Input: part model. Units: mm. Frame: model coordinates. A direction names the side the tool comes from. Coordinates: 2 decimals unless noted, no trailing zeros. Loops run counter-clockwise (first coordinate to the right, second up) from the corner with the lowest first, then second, coordinate; pieces in that order, holes last.
(1) Section C-C, the plane y = 16. Return loops of the section in (x, z), then the cut area to 3 significant figures.
(2) Section D-D, the plane x = 21.5. Return loops of the section in (y, z).
(3) Section B-B, the plane x = 4. Return loops of the section in (y, z).
(4) Line query: L1, parallel to X at y = 6, z = 1.45; L2, parallel to X at y = 10, z = 1.9; L3, parallel to X at y = 73.5, z = 1.55. Output: solid intervals per line, ascending.
(5) Set-up query: faces 4 (the face through (31, 13.53, 1)), 5 (the face through (25, 3.13, 1)), 6 (the face through (21, 37.18, 1)), 7 (the face through (-24, 3.13, 1)), 8 (the face through (38.259, 12, 1)). Return all of +Z, -Z, +X, -X, +Y, -Y with unobstructed straight access to the full face (end or side cutting, diameter ignored); none if empty.
(6) Mould query, pull axis Y, two halves, no side actions, for faces 1 (the face through (-17.563, 34, 1)), 2 (the face through (20.209, 0, 1)), 3 (the face through (-0.165, 90.126, 0.986)). Classes: released by +Y, released by -Y, zero draft, split by the parting line, or undercut.
(7) Contact query for flat-ended pins moving along their axis: P1, Ø0.6, axis at x = -20.5, z = 1, coming from the -Y side; P2, Ø0.6, axis at y = 34.5, z = 1.5, coming from the -X side; P3, Ø1, axis at y = 0.5, z = 1, coming from the +X side. Output: stop coordinate, or through.
(8) Section A-A, the plane y = 5.5. Return loops of the section in (x, z), then the cut area to 3 significant figures.
```python
from build123d import *

# Parameters (mm, degrees)
SKETCH_1_R      = 9.55
SKETCH_1_R_2    = 2.55
SKETCH_1_W      = 6.1
SKETCH_1_H      = 6.1
EXTRUDE_1_DEPTH = 2
FILLET_3_R      = 1.5


with BuildPart() as part:
    # 草图1 → 凸台-拉伸1 (new body)
    with BuildSketch(Plane.XY):
        with BuildLine():
            Line((-28.741188564, 3.13029316), (-28.741188564, 7.13029316))
            Line((-28.741188564, 7.13029316), (-27.291188564, 7.13029316))
            Line((-27.291188564, 7.13029316), (-27.291188564, 10.33029316))
            Line((-27.291188564, 10.33029316), (-28.741188564, 10.33029316))
            Line((-28.741188564, 10.33029316), (-28.741188564, 13.53029316))
            Line((-28.741188564, 13.53029316), (-32.841188564, 13.53029316))
            Line((-32.841188564, 13.53029316), (-32.841188564, 10.33029316))
            Line((-32.841188564, 10.33029316), (-34.291188564, 10.33029316))
            Line((-34.291188564, 10.33029316), (-34.291188564, 7.13029316))
            Line((-34.291188564, 7.13029316), (-32.841188564, 7.13029316))
            Line((-32.841188564, 7.13029316), (-32.841188564, 3.13029316))
            Line((-32.841188564, 3.13029316), (-37.841188564, 3.13029316))
            Line((-37.841188564, 3.13029316), (-37.841188564, 20.08029316))
            Line((-37.841188564, 20.08029316), (-16.791188564, 73.13029316))
            ThreePointArc((-16.791188564, 73.13029316), (0.208811436, 90.13029316), (17.208811436, 73.13029316))
            Line((17.208811436, 73.13029316), (38.258811436, 20.08029316))
            Line((38.258811436, 20.08029316), (38.258811436, 3.13029316))
            Line((38.258811436, 3.13029316), (33.258811436, 3.13029316))
            Line((33.258811436, 3.13029316), (33.258811436, 7.13029316))
            Line((33.258811436, 7.13029316), (34.708811436, 7.13029316))
            Line((34.708811436, 7.13029316), (34.708811436, 10.33029316))
            Line((34.708811436, 10.33029316), (33.258811436, 10.33029316))
            Line((33.258811436, 10.33029316), (33.258811436, 13.53029316))
            Line((33.258811436, 13.53029316), (29.158811436, 13.53029316))
            Line((29.158811436, 13.53029316), (29.158811436, 10.33029316))
            Line((29.158811436, 10.33029316), (27.708811436, 10.33029316))
            Line((27.708811436, 10.33029316), (27.708811436, 7.13029316))
            Line((27.708811436, 7.13029316), (29.158811436, 7.13029316))
            Line((29.158811436, 7.13029316), (29.158811436, 3.13029316))
            Line((29.158811436, 3.13029316), (20.208811436, 3.13029316))
            Line((20.208811436, 3.13029316), (20.208811436, -2.86970684))
            Line((20.208811436, -2.86970684), (12.208811436, -2.86970684))
            Line((12.208811436, -2.86970684), (12.208811436, 3.13029316))
            Line((12.208811436, 3.13029316), (-11.791188564, 3.13029316))
            Line((-11.791188564, 3.13029316), (-11.791188564, -2.86970684))
            Line((-11.791188564, -2.86970684), (-19.791188564, -2.86970684))
            Line((-19.791188564, -2.86970684), (-19.791188564, 3.13029316))
            Line((-19.791188564, 3.13029316), (-28.741188564, 3.13029316))
        make_face()
        with Locations((0.208811436, 73.13029316)):
            Circle(SKETCH_1_R, mode=Mode.SUBTRACT)
        with Locations((-4.791188564, 28.13029316)):
            Circle(SKETCH_1_R_2, mode=Mode.SUBTRACT)
        with Locations(Location((5.208811436, 28.13029316, 0), (0, 0, 180))):
            Circle(SKETCH_1_R_2, mode=Mode.SUBTRACT)
        with Locations((-20.612527992, 34.13029316)):
            Rectangle(SKETCH_1_W, SKETCH_1_H, mode=Mode.SUBTRACT)
        with Locations((-20.612527992, 17.03029316)):
            Rectangle(SKETCH_1_W, SKETCH_1_H, mode=Mode.SUBTRACT)
        Polygon((0.208811436, 22.13029316), (-11.791188564, 10.33029316), (11.812144769, 10.33029316), align=None, mode=Mode.SUBTRACT)
        with Locations((21.030150863, 34.13029316)):
            Rectangle(SKETCH_1_W, SKETCH_1_H, mode=Mode.SUBTRACT)
        with Locations((21.030150863, 17.03029316)):
            Rectangle(SKETCH_1_W, SKETCH_1_H, mode=Mode.SUBTRACT)
        Polygon((0.208811436, 56.417251186), (-10.987657951, 39.784470466), (0.208811436, 37.232850696), (11.405280822, 39.784470466), align=None, mode=Mode.SUBTRACT)
    extrude(amount=EXTRUDE_1_DEPTH)

    # 圆角3
    fillet_3_edges = [part.edges().sort_by_distance(p)[0] for p in [
        (11.405280822, 39.784470466, 1),
        (0.208811436, 56.417251186, 1),
        (-10.987657951, 39.784470466, 1),
        (0.208811436, 37.232850696, 1),
        (11.812144769, 10.33029316, 1),
        (0.208811436, 22.13029316, 1),
        (-11.791188564, 10.33029316, 1),
    ]]
    fillet(fillet_3_edges, radius=FILLET_3_R)


solid = part.part
```
Report:
1. outline: (-37.84, 0) - (-23.66, 0) - (-23.66, 2) - (-37.84, 2) - close; (-17.56, 0) - (-6.03, 0) - (-6.03, 2) - (-17.56, 2) - close; (6.24, 0) - (17.98, 0) - (17.98, 2) - (6.24, 2) - close; (24.08, 0) - (38.26, 0) - (38.26, 2) - (24.08, 2) - close
1. area: 103 mm2
2. outline: (3.13, 0) - (13.98, 0) - (13.98, 2) - (3.13, 2) - close; (20.08, 0) - (31.08, 0) - (31.08, 2) - (20.08, 2) - close; (37.18, 0) - (62.32, 0) - (62.32, 2) - (37.18, 2) - close
3. outline: (3.13, 0) - (10.33, 0) - (10.33, 2) - (3.13, 2) - close; (18.27, 0) - (25.89, 0) - (25.89, 2) - (18.27, 2) - close; (30.38, 0) - (38.1, 0) - (38.1, 2) - (30.38, 2) - close; (50.79, 0) - (64.37, 0) - (64.37, 2) - (50.79, 2) - close; (81.9, 0) - (89.7, 0) - (89.7, 2) - (81.9, 2) - close
4. L1: x = -37.84 to -32.84, -28.74 to 29.16, 33.26 to 38.26
4. L2: x = -37.84 to -34.29, -27.29 to 27.71, 34.71 to 38.26
4. L3: x = -16.79 to -9.33, 9.75 to 17.2
5. face 4: +Z, -Z, -Y
5. face 5: +Z, -Z, +X, -Y
5. face 6: +Z, -Z
5. face 7: +Z, -Z, -X, -Y
5. face 8: +Z, -Z, +X, +Y, -Y
6. face 1: undercut
6. face 2: zero draft
6. face 3: released by +Y
7. P1: stops at y = 3.13
7. P2: stops at x = -32.24
7. P3: stops at x = 20.21
8. outline: (-37.84, 0) - (-32.84, 0) - (-32.84, 2) - (-37.84, 2) - close; (-28.74, 0) - (29.16, 0) - (29.16, 2) - (-28.74, 2) - close; (33.26, 0) - (38.26, 0) - (38.26, 2) - (33.26, 2) - close
8. area: 136 mm2
